Build history of the part. All positions in model axes, mm. Face numbers are marked on the shaded views. A direction names the side the tool comes from. Coordinates: 2 decimals unless noted, no trailing zeros. Order: outer loops, then holes, each group sorted by start corner. A loop starts at its lowest first (then second) coordinate and runs counter-clockwise, first axis right, second up. Notation, with made-up numbers: M -18,26.25 L 33,26.25 A33 ccw 33,59.25 Z; hole C 76.25,10 d5. An arc over 180 degrees is marked long. Write item = value, one per line. Start each with the question number.
Q1. 3-axis set-ups, long thin cutter, end or side, ignore diameter. For the marked faces 4 and 5: which of +Z, -Z, +X, -X, +Y, -Y reach the whole face in a straight line?
Q2. Band-saw the part on B-B on x = -2.5. Write the cut outline in (y, z).
Q3. Drill centre lines: probe 1 along Y at (x, z) = (0, 5.45); probe 2 along Z at (x, y) = (-5.25, 3); probe 3 along X at (y, z) = (-8.75, 0.5). Where is each one in solid material? Low to high.
Q4. Band-saw the part on A-A on y = 4.5. Write the cut outline in (x, z).
Q5. Pull direction X, two halves, no side cores. Call the marked faces 1, 2 and 3: released by +X, released by -X, zero draft, split by the parting line, or undercut.
Q6. Pin check, flat tip, straight feed: P1, Ø3, axis at x = -5, z = 1.5, coming from the -Y side. Stop position of the tip, or through.
Q7. Band-saw the part on C-C on z = 0.6. Write the cut outline in (x, y).
Q8. Band-saw the part on D-D on z = 4. Write the cut outline in (x, y).
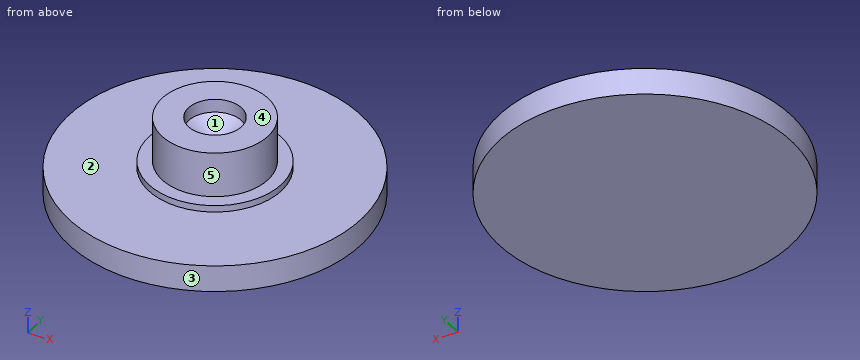
```python
from build123d import *

# Parameters (mm, degrees)
F0_R     = 11
F1_DEPTH = 2
F2_R     = 5
F3_DEPTH = 0.5
F4_R     = 4
F5_DEPTH = 3.4
F7_D     = 4
F7_DEPTH = 1
F7_TIP   = 1.2017212381


with BuildPart() as f1:
    # F0 (on Top) → F1 (new body)
    with BuildSketch(Plane.XY):
        Circle(F0_R)
    extrude(amount=F1_DEPTH)

    # F2 (on face) → F3 (join)
    with BuildSketch(Plane.XY.offset(2)):
        Circle(F2_R)
    extrude(amount=F3_DEPTH)

    # F4 (on face) → F5 (join)
    with BuildSketch(Plane.XY.offset(2.5)):
        Circle(F4_R)
    extrude(amount=F5_DEPTH)

    # F7
    with Locations(Plane.XY.offset(5.9)):
        with Locations((0, 0)):
            Hole(F7_D / 2, depth=F7_DEPTH)
            with Locations((0, 0, -(F7_DEPTH + F7_TIP / 2))):  # 118° drill point
                Cone(0, F7_D / 2, F7_TIP, mode=Mode.SUBTRACT)


solid = f1.part
```
Recorded:
q1.face_4 = +Z, +X, -X, +Y, -Y
q1.face_5 = +Z
q2.outline = M -10.71,0 L 10.71,0 L 10.71,2 L 4.33,2 L 4.33,2.5 L 3.12,2.5 L 3.12,5.9 L -3.12,5.9 L -3.12,2.5 L -4.33,2.5 L -4.33,2 L -10.71,2 Z
q3.probe_1 = -4 to -2, 2 to 4
q3.probe_2 = 0 to 2
q3.probe_3 = -6.67 to 6.67
q4.outline = M -10.04,0 L 10.04,0 L 10.04,2 L 2.18,2 L 2.18,2.5 L -2.18,2.5 L -2.18,2 L -10.04,2 Z
q5.face_1 = undercut
q5.face_2 = zero draft
q5.face_3 = split by the parting line
q6.P1 = -10.43
q7.outline = C 0,0 d22
q8.outline = C 0,0 d8; hole C 0,0 d1
